Build history of the part. All positions in model axes, mm. Face numbers are marked on the shaded views. A direction names the side the tool comes from. Round coordinates to 2 decimals unless told otherwise and drop trailing zeros. Write each loop counter-clockwise with the first axis right and the second up, starting at its lowest first coordinate (ties: lowest second). Pieces come first, ordered by that corner, then holes.
Item 1: Mould opens along X. For the marked faces 3, 4, 5 and 6 say: +X half, -X half, draft (parallel to the pull), parting line (faces both ways), or undercut.
Item 2: Wall check: probe 1 along Z at (x, y) = (-51.5, -6.25); probe 2 along X at (y, z) = (-10.75, -72); probe 3 along X at (y, z) = (-12.25, -4). Give the ranges that are in metal, low to high.
Item 3: Band-saw the part on A-A, the plane z = -64. Write the cut outline in (x, y), then the cut area to 3 significant figures.
Item 4: Band-saw the part on C-C, the plane y = -9. Write the cut outline in (x, z).
Item 5: Band-saw the part on B-B, the plane x = 51.5. Write the cut outline in (y, z), then the cut area to 3 significant figures.
Item 6: Band-saw the part on D-D, the plane z = -40. Count the separate pieces of the cut face and the enclosed holes in it, then the cut area to 3 significant figures.
Item 7: 3-axis set-ups, long thin cutter, end or side, ignore diameter. For the marked faces 1 and 2: which of +Z, -Z, +X, -X, +Y, -Y reach the whole face in a straight line?
Solid Edge part; units mm, degrees
sketch "Sketch1" plane through (0, 0, 0) normal (0, -1, 0) x (1, 0, 0)
  line L0 (59, 0) -> (-59, 0)
  line L1 (-59, 0) -> (-59, -80)
  line L2 (-59, -80) -> (59, -80)
  line L3 (59, -80) -> (59, 0)
extrude "Protrusion1" add sketch "Sketch1" along normal blind 15
sketch "Sketch2" plane through (0, 0, 0) normal (0, -1, 0) x (1, 0, 0)
  line L0 (-44, -30) -> (44, -30)
  line L1 (44, -30) -> (44, -110)
  line L2 (44, -110) -> (-44, -110)
  line L3 (-44, -110) -> (-44, -30)
extrude "Extrusionsausschnitt_1" cut sketch "Sketch2" along normal mid plane 380
fillet "Verrundung_1" radius 30 2 edges at (-44, -7.5, -30) (44, -7.5, -30)
hole "Bohrung_2" at (-51.5, -15, -72) direction (0, 1, 0) diameter 6.3 depth 30
hole "Hole1" at (-51.5, -15, -40) direction (0, 1, 0) diameter 6.3 depth 30
hole "Hole2" at (-43, -15, -5) direction (0, 1, 0) diameter 6.3 depth 30
mirror "Mirror1" about plane through (0, 0, 0) normal (1, 0, 0) of "Bohrung_2", "Hole1", "Hole2"
fillet "Verrundung_2" radius 2 6 edges at (-59, -7.5, 0) (-59, -7.5, -80) (-44, -7.5, -80) (44, -7.5, -80) (59, -7.5, -80) (59, -7.5, 0)
chamfer "Fase_2" distance 0.5 angle 45 22 edges at (51.5, -15, -68.85) (51.5, -15, -36.85) (43, -15, -1.85) (-43, -15, -1.85) (-51.5, -15, -36.85) (-51.5, -15, -68.85) (59, -15, -40) (58.4142, -15, -0.5858) (0, -15, 0) (-58.4142, -15, -0.5858) (-59, -15, -40) (-58.4142, -15, -79.4142) (-51.5, -15, -80) (-44.5858, -15, -79.4142) (-44, -15, -69) (-35.2132, -15, -38.7868) (0, -15, -30) (35.2132, -15, -38.7868) (44, -15, -69) (44.5858, -15, -79.4142) (51.5, -15, -80) (58.4142, -15, -79.4142)
chamfer "Fase_3" distance 0.5 angle 45 22 edges at (51.5, 0, -68.85) (51.5, 0, -36.85) (43, 0, -1.85) (-43, 0, -1.85) (-51.5, 0, -36.85) (-51.5, 0, -68.85) (0, 0, 0) (58.4142, 0, -0.5858) (59, 0, -40) (58.4142, 0, -79.4142) (51.5, 0, -80) (44.5858, 0, -79.4142) (44, 0, -69) (35.2132, 0, -38.7868) (0, 0, -30) (-35.2132, 0, -38.7868) (-44, 0, -69) (-44.5858, 0, -79.4142) (-51.5, 0, -80) (-58.4142, 0, -79.4142) (-59, 0, -40) (-58.4142, 0, -0.5858)
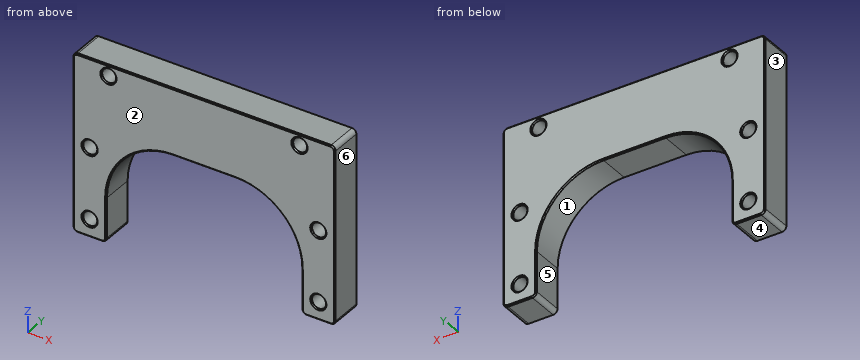
Results:
1. face 3: -X half
1. face 4: draft
1. face 5: undercut
1. face 6: +X half
2. probe 1: z = -80 to -75.15, -68.85 to -43.15, -36.85 to 0
2. probe 2: x = -59 to -54.65, -48.35 to -44, 44 to 48.35, 54.65 to 59
2. probe 3: x = -59 to -45.99, -40.01 to 40.01, 45.99 to 59
3. outline: (-59, -14.5) - (-58.5, -15) - (-44.5, -15) - (-44, -14.5) - (-44, -0.5) - (-44.5, 0) - (-58.5, 0) - (-59, -0.5) - close; (44, -14.5) - (44.5, -15) - (58.5, -15) - (59, -14.5) - (59, -0.5) - (58.5, 0) - (44.5, 0) - (44, -0.5) - close
3. area: 449 mm2
4. outline: (-59, -78) arc R2 ccw to (-57, -80) - (-46, -80) arc R2 ccw to (-44, -78) - (-44, -60) arc R30 cw to (-14, -30) - (14, -30) arc R30 cw to (44, -60) - (44, -78) arc R2 ccw to (46, -80) - (57, -80) arc R2 ccw to (59, -78) - (59, -2) arc R2 ccw to (57, 0) - (-57, 0) arc R2 ccw to (-59, -2) - close; hole circle Ø6.3 at (-51.5, -72); hole circle Ø6.3 at (-51.5, -40); hole circle Ø6.3 at (-43, -5); hole circle Ø6.3 at (43, -5); hole circle Ø6.3 at (51.5, -72); hole circle Ø6.3 at (51.5, -40)
5. outline: (-15, -79.5) - (-14.5, -80) - (-0.5, -80) - (0, -79.5) - (0, -75.65) - (-0.5, -75.15) - (-14.5, -75.15) - (-15, -75.65) - close; (-15, -68.35) - (-14.5, -68.85) - (-0.5, -68.85) - (0, -68.35) - (0, -43.65) - (-0.5, -43.15) - (-14.5, -43.15) - (-15, -43.65) - close; (-15, -36.35) - (-14.5, -36.85) - (-0.5, -36.85) - (0, -36.35) - (0, -0.5) - (-0.5, 0) - (-14.5, 0) - (-15, -0.5) - close
5. area: 1,010 mm2
6. separate pieces: 4
6. enclosed holes: 0
6. area: 488 mm2
7. face 1: -Z, +Y, -Y
7. face 2: +Z, -Z, +X, -X, -Y
